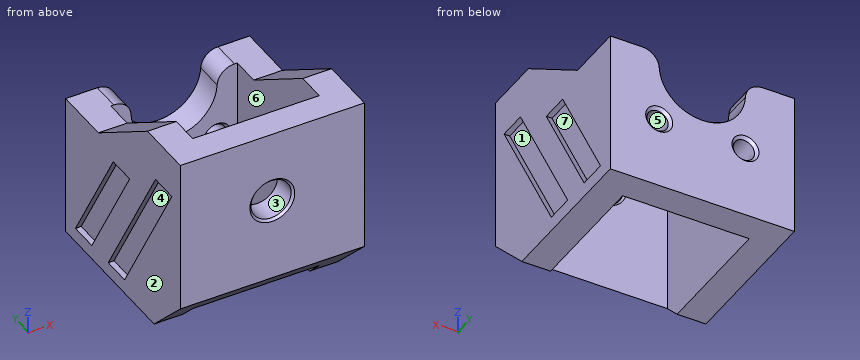
Solid Edge part; units mm, degrees
sketch "Sketch1" plane through (0, 0, 0) normal (0, 0, 1) x (1, 0, 0)
  line L0 (-11, -12.5) -> (11, -12.5)
  line L1 (11, -12.5) -> (11, 12.5)
  line L2 (11, 12.5) -> (-11, 12.5)
  line L3 (-11, 12.5) -> (-11, -12.5)
  line L4 (-16, -17.5) -> (16, -17.5)
  line L5 (16, -17.5) -> (16, 17.5)
  line L6 (16, 17.5) -> (-16, 17.5)
  line L7 (-16, 17.5) -> (-16, -17.5)
  dimension "D1" = 11
  dimension "D2" = 11
extrude "body" add sketch "Sketch1" against normal blind 12.5 and the other way blind 22.5
sketch "Sketch2" plane through (16, 0, 4) normal (1, 0, 0) x (0, 0, -1)
  line L0 (-18.5, 17.5) -> (-8.5, 17.5)
  line L1 (-8.5, 17.5) -> (-8.5, 7.5)
  line L2 (-8.5, 7.5) -> (-18.5, -7.5)
  line L3 (-18.5, -7.5) -> (-18.5, 17.5)
  dimension "D1" = 18.5
  dimension "D2" = 8.5
extrude "Cutout1" cut sketch "Sketch2" against normal through all
chamfer "side_chamfer" distance 8 angle 45 1 edges at (0, -17.5, -12.5)
hole "Hole1" at (-7.5, 17.5, 0) direction (0, -1, 0) diameter 3.7 depth 10 tip angle 118 start chamfer 0.5 start chamfer angle 45 end chamfer 0.5 end chamfer angle 45
hole "Hole2" at (7.5, 17.5, 0) direction (0, -1, 0) diameter 3.7 depth 10 tip angle 118 start chamfer 0.5 start chamfer angle 45 end chamfer 0.5 end chamfer angle 45
sketch "Sketch3" plane through (-16, 0, 5) normal (-1, 0, 0) x (0, 0, 1)
  line L0 (-15, 14.5) -> (-15, 9.5)
  line L1 (-15, 9.5) -> (5, -2.047)
  line L2 (5, -2.047) -> (5, 2.953)
  line L3 (5, 2.953) -> (-15, 14.5)
  line L4 (-15, 4.5) -> (-15, -0.5)
  line L5 (-15, -0.5) -> (10, -14.9338)
  line L6 (10, -9.9338) -> (10, -14.9338)
  line L7 (-15, 4.5) -> (10, -9.9338)
  dimension "D1" = 15
  dimension "D2" = 5
  dimension "D3" = 15
  dimension "D4" = 15
extrude "design_cutout" cut sketch "Sketch3" against normal blind 1
hole "leg_screw_cutout" at (0, -12.5, 10) direction (0, -1, 0) diameter 7 end up to next start chamfer 0.4 start chamfer angle 45 end chamfer 0.4 end chamfer angle 45
sketch "Sketch4" plane through (0, 17.5, 0) normal (0, 1, 0) x (0, 0, -1)
  circle A0 centre (-10, 0) radius 7.5
extrude "Cutout2" cut sketch "Sketch4" against normal up to next
fillet "screw_helper_rounding" radius 3 2 edges at (-7.0711, 15, 12.5) (7.0711, 15, 12.5)
mirror "Mirror1" about plane through (0, 0, 0) normal (1, 0, 0) of "design_cutout"
properties material "Polyethylene, low density"
Model file for the job. Use its own axes, mm. Face numbers are marked on the shaded views. A direction names the side the tool comes from. Coordinates: 2 decimals unless noted, no trailing zeros. Loops run counter-clockwise (first coordinate to the right, second up) from the corner with the lowest first, then second, coordinate; pieces in that order, holes last. Notation, with made-up numbers: (-11.75, 50.25) - (3.25, 50.25) arc R27 ccw to (3.25, 76.25) - close; hole circle Ø8 at (53.5, 3). An arc over 180 degrees is marked (long way). Answer as a JSON object with one key per item and string values. Group by question number.
(1) Flat gauge pins, fed straight in: pin 1 (4.5 mm diameter, centred on x = -12, y = 11.5, fed in from +Z); pin 2 (6 mm diameter, centred on x = -3, y = 7, fed in from +Z); pin 3 (2 mm diameter, centred on x = 4, z = 16, fed in from +Y); pin 4 (1.1 mm diameter, centred on x = 15.5, y = 1, fed in from +Z). Where does each tip first touch, or does it go through?
(2) Two-plate mould, pull along X, no slides. Class the marked faces 1, 2 and 3: released by +X, released by -X, zero draft, split by the parting line, or undercut.
(3) Cut at B-B (y = -8). Give the cut face in (x, z), then the cut area to 3 significant figures.
(4) Probe line 1 along X through (y, z) = (15.65, 0); line 2 along X through (y, z) = (1, 16); line 3 along X through (y, z) = (-8, 7.5). List the from-to ranges inside material, lowest first.
(5) Tool access for the marked faces 4, 5, 6 and 7: list every direction of +Z, -Z, +X, -X, +Y, -Y with a clear straight run to the whole face (end or side of a thin tool).
(6) Cut at D-D (y = 15.5). Give the cut face in (x, z), then the cut area to 3 significant figures.
(7) Cut at A-A (x = -4.5). Give the cut face in (y, z), then the cut area to 3 significant figures.
(8) Cut at C-C (x = 0). Give the cut face in (y, z), then the cut area to 3 significant figures.
Geometry says:
{
 "1": {"pin 1": "stops at z = 12.5", "pin 2": "passes through", "pin 3": "stops at y = -12.5", "pin 4": "stops at z = 17.2"},
 "2": {"face 1": "released by +X", "face 2": "released by -X", "face 3": "undercut"},
 "3": {"outline": "(-16, -12.5) - (-11, -12.5) - (-11, 22.5) - (-16, 22.5) - (-16, 11.65) - (-15, 11.65) - (-15, 2.99) - (-16, 2.99) - close; (11, -12.5) - (16, -12.5) - (16, 2.99) - (15, 2.99) - (15, 11.65) - (16, 11.65) - (16, 22.5) - (11, 22.5) - close", "area": "333 mm^2"},
 "4": {"line 1": "x = -16 to -9.35, -5.65 to 5.65, 9.35 to 16", "line 2": "x = -16 to -11, 11 to 16", "line 3": "x = -15 to -11, 11 to 15"},
 "5": {"face 4": "-X", "face 5": "+Y", "face 6": "+Z, -Z", "face 7": "+X"},
 "6": {"outline": "(-16, -12.5) - (16, -12.5) - (16, 12.5) - (10.49, 12.5) arc R3 ccw to (7.49, 9.64) arc R7.5 cw to (-7.49, 9.64) arc R3 ccw to (-10.49, 12.5) - (-16, 12.5) - close; hole circle Ø3.7 at (-7.5, 0); hole circle Ø3.7 at (7.5, 0)", "area": "649 mm^2"},
 "7": {"outline": "(-17.5, -4.5) - (-12.5, -9.5) - (-12.5, 22.5) - (-17.5, 22.5) - close; (12.5, -12.5) - (17.5, -12.5) - (17.5, 4) - (12.5, 4) - close", "area": "230 mm^2"},
 "8": {"outline": "(-17.5, -4.5) - (-12.5, -9.5) - (-12.5, 6.1) - (-12.9, 6.5) - (-17.1, 6.5) - (-17.5, 6.1) - close; (-17.5, 13.9) - (-17.1, 13.5) - (-12.9, 13.5) - (-12.5, 13.9) - (-12.5, 22.5) - (-17.5, 22.5) - close; (12.5, -12.5) - (17.5, -12.5) - (17.5, 2.5) - (12.5, 2.5) - close", "area": "187 mm^2"}
}
